from build123d import *

# Parameters (mm, degrees)
SKETCH_W             = 25.4
SKETCH_H             = 3.175
PAD_DEPTH            = 25.4
SKETCH001_W          = 28.575
SKETCH001_H          = 12.7
PAD001_DEPTH         = 1.81
PAD001_DEPTH_BACK    = 5.715
POCKET_DEPTH         = 9.525
POCKET001_DEPTH      = 12.7
CHAMFER_SIZE         = 1.8034
SKETCH004_R          = 3.2512
POCKET002_DEPTH      = 5.716
PAD002_DEPTH         = 10.795
FILLET_R             = 4.953
SKETCH013_W          = 9.37
SKETCH013_H          = 12.7
SKETCH013_R          = 1.6002
PAD008_DEPTH         = 20.955
POCKET003_DEPTH      = 11.3711
SKETCH014_W          = 2.825
SKETCH014_H          = 10.1538
POCKET004_DEPTH      = 5.6125
SKETCH015_W          = 2.825
SKETCH015_H          = 5.725
POCKET005_DEPTH      = 7.8269
SKETCH016_R          = 0.6125
SKETCH016_W          = 0.65
SKETCH016_H          = 0.225
POCKET006_DEPTH      = 6.6241
SKETCH017_R          = 0.6125
SKETCH017_W          = 0.65
SKETCH017_H          = 0.225
POCKET007_DEPTH      = 7.6241
POCKET007_DEPTH_BACK = 20.9529
SKETCH018_R          = 1.6002
SKETCH019_R          = 2.36517
SKETCH020_W          = 25.4
SKETCH020_H          = 6.35
POCKET008_DEPTH      = 2.54
FILLET001_R          = 2.286


with BuildPart() as part:
    # Sketch → Pad (new body)
    with BuildSketch(Plane.XY):
        with Locations((-12.7, 1.5875)):
            Rectangle(SKETCH_W, SKETCH_H)
    extrude(amount=PAD_DEPTH)

    # Sketch001 (on Face1 of Pad) → Pad001 (join, two sides)
    with BuildSketch(Plane(origin=(0, 3.175, 0), x_dir=(-1, 0, 0), z_dir=(0, 1, 0))) as pad001_sk:
        with Locations((-14.2875, 12.7)):
            Rectangle(SKETCH001_W, SKETCH001_H)
    extrude(amount=PAD001_DEPTH)
    extrude(pad001_sk.sketch, amount=-PAD001_DEPTH_BACK)

    # Sketch002 (on Face13 of Pad001) → Pocket (cut)
    with BuildSketch(Plane.YZ.offset(28.575)):
        Polygon((9.150137, 19.05), (2.800137, 12.7), (9.150137, 6.35), align=None)
    extrude(amount=-POCKET_DEPTH, mode=Mode.SUBTRACT)

    # Sketch003 (on Face16 of Pocket) → Pocket001 (cut)
    with BuildSketch(Plane.YZ.offset(19.05)):
        with BuildLine():
            ThreePointArc((4.08, 14.732), (2.048, 12.7), (4.08, 10.668))
            Line((4.985, 10.668), (4.08, 10.668))
            Line((4.985, 14.732), (4.985, 10.668))
            Line((4.08, 14.732), (4.985, 14.732))
        make_face()
    extrude(amount=-POCKET001_DEPTH, mode=Mode.SUBTRACT)

    # Chamfer
    chamfer_edges = [part.edges().sort_by_distance(p)[0] for p in [
        (0, 4.985, 12.7),
    ]]
    chamfer(chamfer_edges, length=CHAMFER_SIZE)

    # Sketch004 (on Face4 of Chamfer) → Pocket002 (cut, through all)
    with BuildSketch(Plane(origin=(0, 3.175, 0), x_dir=(-1, 0, 0), z_dir=(0, 1, 0))):
        with Locations((12.7, 12.7)):
            Circle(SKETCH004_R)
    extrude(amount=-POCKET002_DEPTH, mode=Mode.SUBTRACT)

    # Sketch006 (on Face4 of Pocket002) → Pad002 (join)
    with BuildSketch(Plane(origin=(0, 3.175, 0), x_dir=(-1, 0, 0), z_dir=(0, 1, 0))):
        Polygon((0, 0), (-3.175, 0), (-3.175, 28.575), (25.4, 28.575), (25.4, 25.4), (0, 25.4), align=None)
    extrude(amount=-PAD002_DEPTH)

    # Fillet
    fillet_edges = [part.edges().sort_by_distance(p)[0] for p in [
        (3.175, -2.54, 12.7),
    ]]
    fillet(fillet_edges, radius=FILLET_R)

    # Sketch013 (on Face4 of Fillet) → Pad008 (join)
    with BuildSketch(Plane.YZ.offset(28.575)):
        with Locations((2.145, 12.7)):
            Rectangle(SKETCH013_W, SKETCH013_H)
        with Locations((4.08, 12.7)):
            Circle(SKETCH013_R, mode=Mode.SUBTRACT)
    extrude(amount=PAD008_DEPTH)

    # Pad008 Face13 → Pocket003 (cut)
    with BuildSketch(Plane(origin=(28.575, 5.919165, 12.7), x_dir=(0, 1, 0), z_dir=(-1, 0, 0))):
        with BuildLine():
            Line((-0.934165, -2.184863), (-0.934165, -6.35))
            Line((-0.934165, -6.35), (0.910835, -6.35))
            Line((0.910835, -6.35), (0.910835, 6.35))
            Line((0.910835, 6.35), (-0.934165, 6.35))
            Line((-0.934165, 6.35), (-0.934165, 2.184863))
            Line((-0.934165, 2.184863), (-1.545926, 1.573102))
            ThreePointArc((-1.545926, 1.573102), (-0.608336, 1.022594), (-0.238965, 0))
            ThreePointArc((-0.238965, 0), (-0.608336, -1.022594), (-1.545926, -1.573102))
            Line((-1.545926, -1.573102), (-0.934165, -2.184863))
        make_face()
    extrude(amount=-POCKET003_DEPTH, mode=Mode.SUBTRACT)

    # Sketch014 (on Face15 of Pocket003) → Pocket004 (cut)
    with BuildSketch(Plane(origin=(0, 6.83, 0), x_dir=(-1, 0, 0), z_dir=(0, 1, 0))):
        with Locations((-46.325, 12.7)):
            Rectangle(SKETCH014_W, SKETCH014_H)
    extrude(amount=-POCKET004_DEPTH, mode=Mode.SUBTRACT)

    # Sketch015 (on Face15 of Pocket004) → Pocket005 (cut)
    with BuildSketch(Plane(origin=(0, 6.83, 0), x_dir=(-1, 0, 0), z_dir=(0, 1, 0))):
        with Locations((-43.15, 12.7)):
            Rectangle(SKETCH015_W, SKETCH015_H)
    extrude(amount=-POCKET005_DEPTH, mode=Mode.SUBTRACT)

    # Sketch016 (on Face53 of Pocket005) → Pocket006 (cut, through all)
    with BuildSketch(Plane(origin=(0, -0.9969, 0), x_dir=(-1, 0, 0), z_dir=(0, 1, 0))):
        with Locations((-42.4, 12.7)):
            Circle(SKETCH016_R)
        with Locations((-44.15, 14.975)):
            Rectangle(SKETCH016_W, SKETCH016_H)
        with Locations((-44.15, 10.425)):
            Rectangle(SKETCH016_W, SKETCH016_H)
        with Locations((-42.15, 14.975)):
            Rectangle(SKETCH016_W, SKETCH016_H)
        with Locations((-42.15, 10.425)):
            Rectangle(SKETCH016_W, SKETCH016_H)
    extrude(amount=-POCKET006_DEPTH, mode=Mode.SUBTRACT)

    # Sketch017 (on Face52 of Pocket006) → Pocket007 (cut, two sides)
    with BuildSketch(Plane.XY.offset(7.6231)) as pocket007_sk:
        with Locations((45.575, 4.07924)):
            Circle(SKETCH017_R)
        with Locations((45.325, 6.35424)):
            Rectangle(SKETCH017_W, SKETCH017_H)
        with Locations((45.325, 1.80424)):
            Rectangle(SKETCH017_W, SKETCH017_H)
        with Locations((47.325, 6.35424)):
            Rectangle(SKETCH017_W, SKETCH017_H)
        with Locations((47.325, 1.80424)):
            Rectangle(SKETCH017_W, SKETCH017_H)
    extrude(amount=-POCKET007_DEPTH, mode=Mode.SUBTRACT)
    extrude(pocket007_sk.sketch, amount=POCKET007_DEPTH_BACK, mode=Mode.SUBTRACT)

    # Sketch018 (on Face12 of Pocket007) → SubtractiveLoft section 0
    with BuildSketch(Plane(origin=(39.9461, 0, 0), x_dir=(0, -1, 0), z_dir=(-1, 0, 0))):
        with Locations((-4.07924, 12.7)):
            Circle(SKETCH018_R)
    # Sketch019 (on Face80 of Pocket007) → SubtractiveLoft section 1
    with BuildSketch(Plane.YZ.offset(28.575)):
        with Locations((4.07924, 12.7)):
            Circle(SKETCH019_R)
    loft(mode=Mode.SUBTRACT)

    # Sketch020 (on Face2 of SubtractiveLoft) → Pocket008 (cut)
    with BuildSketch(Plane.XZ.offset(2.54)):
        with Locations((24.003, 12.7)):
            Rectangle(SKETCH020_W, SKETCH020_H)
    extrude(amount=-POCKET008_DEPTH, mode=Mode.SUBTRACT)

    # Fillet001
    fillet001_edges = [part.edges().sort_by_distance(p)[0] for p in [
        (24.003, 0, 15.875),
        (36.703, 0, 12.7),
        (24.003, 0, 9.525),
        (11.303, 0, 12.7),
    ]]
    fillet(fillet001_edges, radius=FILLET001_R)


solid = part.part
Could you check a few things on this model? Use its own coordinates, in mm. A direction names the side the tool comes from. Give positions to 0.01 mm unless a question says otherwise; leave off trailing zeros. Order: outer loops, then holes, each group sorted by start corner. A loop starts at its lowest first (then second) coordinate and runs counter-clockwise, first axis right, second up.
1. Suppose I cut it at A-A (x = 15). List the corners of the cut face in (y, z) for me (3 decimals).
2. We'd pull the mould along Y, two halves only. Please class faces 1 (the flat face through (-13, -4, 25.4)), 2 (the flat face through (46, 1.218, 13)), 3 (the cylindrical face through (48.62, 3.73, 11.14)): pulls with the +Y half, pulls with the -Y half, needs draft (parallel to the pull), parting line crosses it, or undercut.
3. I need wall thicknesses on L1, parallel to Z at x = 41.25, y = 4.08; L2, parallel to Z at x = 44, y = 4; L3, parallel to X at y = 2.75, z = 23.25 (3 decimals). Which ranges of each line are inside material? Lowest first, please.
4. Suppose I cut it at C-C (y = -3.25). List the corners of the cut face in (x, z) for me (3 decimals).
5. For faces 4 (the cylindrical face through (4.664, -3.952, 12.789)), 5 (the cylindrical face through (44.74, 3.73, 11.14)), 6 (the flat face through (41.738, 2, 13)), 7 (the cylindrical face through (11.7, -1, 12.7)), 8 (the flat face through (-25.4, 1, 17)), which set-ups out of +Z, -Z, +X, -X, +Y, -Y let a thin tool reach every point of the face, with its end or its side?
6. Will these pins go through, and if not, where does the flat tip stop? P1, Ø2.5, axis at x = 43.5, y = 3, coming from the +Z side; P2, Ø6, axis at y = -5, z = 12, coming from the -X side; P3, Ø1, axis at y = -5, z = 13.5, coming from the +X side.
7. Suppose I cut it at D-D (x = -20). List the corners of the cut face in (y, z) for me (3 decimals), plus the area to 3 significant figures.
8. Suppose I cut it at B-B (z = 21). List the corners of the cut face in (x, y) for me (3 decimals).
Solved:
1. outline: (-2.54, 6.35) - (4.985, 6.35) - (4.985, 10.668) - (4.08, 10.668) arc R2.032 cw to (4.08, 14.732) - (4.985, 14.732) - (4.985, 19.05) - (-2.54, 19.05) - (-2.54, 15.875) - (-2.286, 15.875) arc R2.286 cw to (0, 13.589) - (0, 11.811) arc R2.286 cw to (-2.286, 9.525) - (-2.54, 9.525) - close
2. face 1: needs draft
2. face 2: pulls with the +Y half
2. face 3: undercut
3. L1: z = 6.35 to 11.1, 14.3 to 19.05
3. L2: z = 6.35 to 9.84, 15.56 to 19.05
3. L3: x = -25.4 to 3.175
4. outline: (-25.4, 25.4) - (0, 25.4) - (0, 0) - (3.175, 0) - (3.175, 6.35) - (5.573, 6.35) - (5.573, 19.05) - (3.175, 19.05) - (3.175, 28.575) - (-25.4, 28.575) - close
5. face 4: +Z, -Z, +X, -Y
5. face 5: +X
5. face 6: +Y
5. face 7: -Y
5. face 8: +Z, -Z, -X, +Y, -Y
6. P1: stops at z = 19.05
6. P2: stops at x = 0
6. P3: stops at x = 4.18
7. outline: (-7.62, 25.4) - (0, 25.4) - (0, 0) - (3.175, 0) - (3.175, 28.575) - (-7.62, 28.575) - close
7. area: 115 mm2
8. outline: (-25.4, 0) - (0, 0) - (0, -7.62) - (3.175, -7.62) - (3.175, 3.175) - (-25.4, 3.175) - close
